Could you check a few things on this model? Use its own coordinates, in mm. Face numbers are marked on the shaded views. A direction names the side the tool comes from. Round coordinates to 2 decimals unless told otherwise and drop trailing zeros. Order: outer loops, then holes, each group sorted by start corner. A loop starts at its lowest first (then second) coordinate and runs counter-clockwise, first axis right, second up. Notation, with made-up numbers: M 75.5,-13.5 L 118.5,-13.5 A24 cw 118.5,4.5 Z; hole C 66.25,63.25 d11. An arc over 180 degrees is marked long. Write each question's results on one line, items separated by ' | '. Start each with the question number.
1. Suppose I cut it at C-C on x = 10. Write out the boundary of the cut face in (y, z), and give its area (3 significant figures).
2. Suppose I cut it at B-B on z = 23. Write out the boundary of the cut face in (x, y).
3. Suppose I cut it at D-D on y = 8. Write out the boundary of the cut face in (x, z).
4. I'm going to push flat-ended pins straight in: pin 1 (5.5 mm diameter, centred on x = 12, z = 35, fed in from -Y); pin 2 (3.5 mm diameter, centred on x = 3, z = 23, fed in from +Y); pin 3 (1.5 mm diameter, centred on x = 8.5, z = 23.5, fed in from +Y). Where does each tip first touch, or does it pass through?
5. For the marked faces 5, 6 and 7, which set-ups out of +Z, -Z, +X, -X, +Y, -Y let a thin tool reach every point of the face, with its end or its side?
6. Suppose I cut it at A-A on y = 0.75. Write out the boundary of the cut face in (x, z), and give its area (3 significant figures).
7. We'd pull the mould along Z, two halves only. Please class the marked faces 1, 2, 3 and 4: released by +Z, released by -Z, zero draft, split by the parting line, or undercut.
8. Please list where these lines run through material, in increasing order: L1, parallel to Z at x = 2, y = 10.5; L2, parallel to Z at x = 7, y = 0.5; L3, parallel to X at y = 1.5, z = 35.
Autodesk Inventor part; units mm, degrees
ref_plane "YZ Plane" through (0, 0, 0) normal (1, 0, 0) x (0, 1, 0)
ref_plane "XZ Plane" through (0, 0, 0) normal (0, 1, 0) x (-1, 0, 0)
ref_plane "XY Plane" through (0, 0, 0) normal (0, 0, 1) x (1, 0, 0)
sketch "Sketch1" plane through (0, 0, 0) normal (0, 0, 1) x (1, 0, 0)
  line L0 (0, 0) -> (20, 0)
  line L1 (20, 0) -> (20, 12)
  line L2 (20, 12) -> (0, 12) construction
  line L3 (0, 12) -> (0, 0)
  arc A0 (2.6515, 12) -> (17.3485, 12) centre (10, 10.5) ccw
  line L4 (0, 12) -> (2.6515, 12)
  line L5 (17.3485, 12) -> (20, 12)
  point P0 (10, 12)
  dimension "d0" = 20
  dimension "d1" = 12
  dimension "d2" = 15
  dimension "d14" = 1.5
extrude "Extrusion1" add sketch "Sketch1" along normal blind 60
sketch "Sketch4" plane through (0, 12, 0) normal (0, 1, 0) x (1, 0, 0)
  line L0 (0, -20) -> (20, -20)
  line L1 (20, -20) -> (20, -40)
  line L2 (20, -40) -> (0, -40)
  line L3 (0, -40) -> (0, -20)
  line L4 (0, 0) -> (0, -60)
  line L5 (17.5, 0) -> (2.5, 0)
  line L6 (20, 0) -> (20, -60)
  point P0 (0, -30)
  point P1 (0, -30)
  point P2 (10, -20)
  point P3 (10, 0)
  point P4 (17.3485, 0)
  point P5 (2.6515, 0)
  dimension "d15" = 20
extrude "Extrusion4" cut sketch "Sketch4" against normal blind 8
sketch "Sketch5" plane through (0, 4, 0) normal (0, 1, 0) x (1, 0, 0)
  circle A0 centre (3, -23) radius 1.6
  circle A1 centre (17, -37) radius 1.6
  line L0 (17, -37) -> (3, -37) construction
  line L1 (3, -37) -> (3, -23) construction
  line L2 (3, -23) -> (17, -23) construction
  line L3 (17, -23) -> (17, -37) construction
  line L4 (0, -40) -> (0, -20) construction
  line L5 (17.5, 0) -> (2.5, 0) construction
  line L6 (6.2583, -40) -> (2.5, -40) construction
  circle A2 centre (12, -35) radius 1.6 construction
  circle A3 centre (12, -35) radius 3
  point P0 (0, 0)
  point P1 (3, -30)
  point P2 (0, -30)
  point P3 (10, -23)
  point P4 (10, 0)
  point P5 (17.3485, 0)
  point P6 (2.6515, 0)
  point P7 (17.3485, -40)
  point P8 (2.6515, -40)
  dimension "d19" = 3.2
  dimension "d20" = 3.2
  dimension "d21" = 3
  dimension "d22" = 3
  dimension "d30" = 6
extrude "Extrusion5" cut sketch "Sketch5" against normal blind 10
sketch "Sketch6" plane through (0, 0, 0) normal (-1, 0, 0) x (0, 0, 1)
  line L0 (7, 0) -> (13, 0)
  line L1 (13, 0) -> (13, 1.5)
  line L2 (13, 1.5) -> (7, 1.5)
  line L3 (7, 1.5) -> (7, 0)
  line L4 (47, 0) -> (53, 0)
  line L5 (53, 0) -> (53, 1.5)
  line L6 (53, 1.5) -> (47, 1.5)
  line L7 (47, 1.5) -> (47, 0)
  line L8 (0, 12) -> (20, 12) construction
  line L9 (40, 12) -> (60, 12) construction
  point P0 (0, 0)
  point P1 (10, 1.5)
  point P2 (10, 12)
  point P3 (50, 1.5)
  point P4 (50, 12)
  dimension "d25" = 6
  dimension "d26" = 1.5
  dimension "d27" = 6
extrude "Extrusion6" cut sketch "Sketch6" against normal through all
equation "\"d20\" = d19"
properties part number "Linear bearing 8mm clamp"
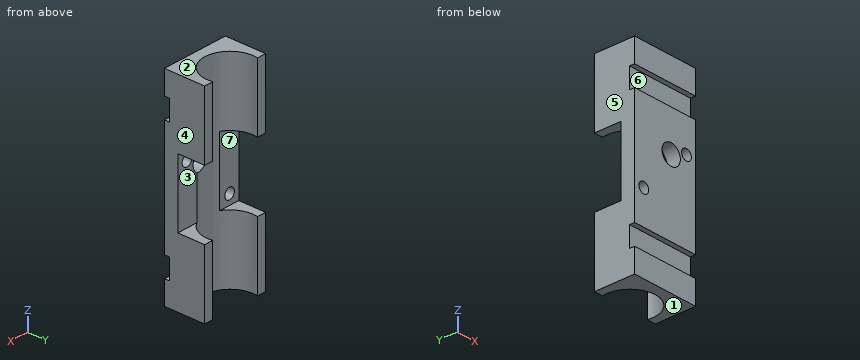
Filled sheet:
1) outline: M 0,0 L 3,0 L 3,32.76 L 0,32.76 L 0,13 L 1.5,13 L 1.5,7 L 0,7 Z; M 0,37.24 L 3,37.24 L 3,60 L 0,60 L 0,53 L 1.5,53 L 1.5,47 L 0,47 Z | area: 149 mm^2
2) outline: M 0,0 L 1.4,0 L 1.4,4 L 0,4 Z; M 4.6,0 L 20,0 L 20,4 L 13.74,4 A7.5 cw 6.26,4 L 4.6,4 Z
3) outline: M 0,0 L 2.93,0 L 2.93,20 L 0,20 Z; M 0,40 L 2.93,40 L 2.93,60 L 0,60 Z; M 17.07,0 L 20,0 L 20,20 L 17.07,20 Z; M 17.07,40 L 20,40 L 20,60 L 17.07,60 Z
4) pin 1: passes through | pin 2: stops at y = 4 | pin 3: stops at y = 3.35
5) face 5: +Z, -Z, -X, +Y, -Y | face 6: +X, -X, -Y | face 7: +X, -X, +Y
6) outline: M 0,0 L 20,0 L 20,7 L 0,7 Z; M 0,13 L 20,13 L 20,47 L 0,47 Z; M 0,53 L 20,53 L 20,60 L 0,60 Z; hole C 3,23 d3.2; hole C 12,35 d6; hole C 17,37 d3.2 | area: 916 mm^2
7) face 1: released by -Z | face 2: released by +Z | face 3: undercut | face 4: zero draft
8) L1: z = 0 to 20, 40 to 60 | L2: z = 0 to 7, 13 to 47, 53 to 60 | L3: x = 0 to 9, 15 to 20
